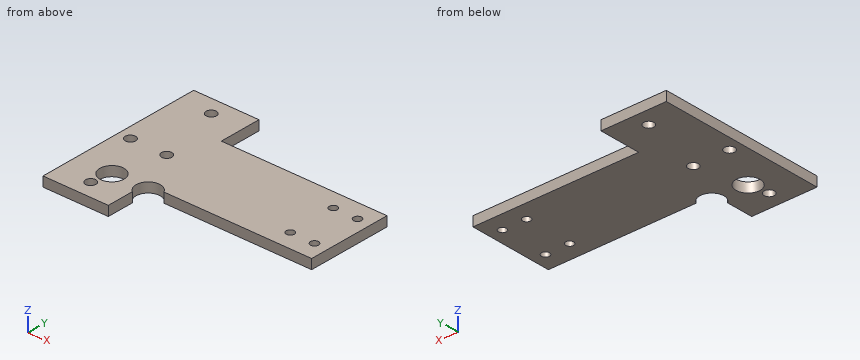
```python
from build123d import *

# Parameters (mm, degrees)
SKETCH_1_W          = 100
SKETCH_1_H          = 35
EXTRUDE_1_DEPTH     = 4
SKETCH_2_R          = 1.65
CUT_EXTRUDE_1_DEPTH = 107.023582282
SKETCH_4_R          = 2.15
CUT_EXTRUDE_3_DEPTH = 107.023582282
SKETCH_8_W          = 27
SKETCH_8_H          = 70
SKETCH_8_R          = 2.15
EXTRUDE_2_DEPTH     = 4
SKETCH_9_R          = 5
CUT_EXTRUDE_6_DEPTH = 4
SKETCH_10_R         = 1.65
CUT_EXTRUDE_7_DEPTH = 10
SKETCH_11_W         = 4.5
SKETCH_11_H         = 35
CUT_EXTRUDE_8_DEPTH = 10


with BuildPart() as part:
    # 草图1 → 凸台-拉伸1 (new body)
    with BuildSketch(Plane.XY):
        with Locations((50, -17.5)):
            Rectangle(SKETCH_1_W, SKETCH_1_H)
    extrude(amount=EXTRUDE_1_DEPTH)

    # 草图2 → 切除-拉伸1 (cut, through all)
    with BuildSketch(Plane.XY.offset(4)):
        with Locations((80, -7.5)):
            Circle(SKETCH_2_R)
        with Locations(Location((80, -27.5, 0), (0, 0, 180))):
            Circle(SKETCH_2_R)
    extrude(amount=-CUT_EXTRUDE_1_DEPTH, mode=Mode.SUBTRACT)

    # 草图4 → 切除-拉伸3 (cut, through all)
    with BuildSketch(Plane.XY.offset(4)):
        with Locations((5, -17.5)):
            Circle(SKETCH_4_R)
        with Locations((20, -17.5)):
            Circle(SKETCH_4_R)
    extrude(amount=-CUT_EXTRUDE_3_DEPTH, mode=Mode.SUBTRACT)

    # 草图8 → 凸台-拉伸2 (add)
    with BuildSketch(Plane.XY.offset(4)):
        with Locations((13.5, -17.5)):
            Rectangle(SKETCH_8_W, SKETCH_8_H)
        with Locations((13.5, 10.5)):
            Circle(SKETCH_8_R, mode=Mode.SUBTRACT)
        with Locations(Location((13.5, -45.5, 0), (0, 0, 180))):
            Circle(SKETCH_8_R, mode=Mode.SUBTRACT)
        with Locations((5, -17.5)):
            Circle(SKETCH_8_R, mode=Mode.SUBTRACT)
        with Locations((20, -17.5)):
            Circle(SKETCH_8_R, mode=Mode.SUBTRACT)
    extrude(amount=-EXTRUDE_2_DEPTH)

    # 草图9 → 切除-拉伸6 (cut)
    with BuildSketch(Plane.XY.offset(4)):
        with Locations((30, -37.34)):
            Circle(SKETCH_9_R)
        with Locations((15, -37.34)):
            Circle(SKETCH_9_R)
    extrude(amount=-CUT_EXTRUDE_6_DEPTH, mode=Mode.SUBTRACT)

    # 草图10 → 切除-拉伸7 (cut)
    with BuildSketch(Plane.XY.offset(4)):
        with Locations((90, -7.5)):
            Circle(SKETCH_10_R)
        with Locations((90, -27.5)):
            Circle(SKETCH_10_R)
    extrude(amount=-CUT_EXTRUDE_7_DEPTH, mode=Mode.SUBTRACT)

    # 草图11 → 切除-拉伸8 (cut)
    with BuildSketch(Plane.XY.offset(4)):
        with Locations((97.75, -17.5)):
            Rectangle(SKETCH_11_W, SKETCH_11_H)
    extrude(amount=-CUT_EXTRUDE_8_DEPTH, mode=Mode.SUBTRACT)


solid = part.part
```
Can you work these out from the model? Positions are in its coordinate system, mm. Round coordinates to 2 decimals unless told otherwise and drop trailing zeros. Loops run counter-clockwise (first coordinate to the right, second up) from the corner with the lowest first, then second, coordinate; pieces in that order, holes last. Notation, with made-up numbers: M -28.5,42 L 25.5,42 A31 ccw 25.5,70 Z; hole C 42,7 d4. An arc over 180 degrees is marked long. Answer as a JSON object with one key per item and string values. Group by question number.
Q1. Imagine slicing it at A-A, the plane x = 5. Please give me the cut outline in (y, z).
Q2. Imagine slicing it at D-D, the plane y = -45.5. Please give me the cut outline in (x, z).
Q3. Please list where these lines run through material, in increasing order: L1, parallel to Y at x = 80, z = 0.6; L2, parallel to X at y = -45.5, z = 0.85; L3, parallel to Y at x = 5, z = 1.95.
Q4. Will these pins go through, and if not, where does the flat tip stop? pin 1 (1.2 mm diameter, centred on x = 54, z = 1, fed in from -Y); pin 2 (3.5 mm diameter, centred on x = 13.5, y = 10.5, fed in from -Z); pin 3 (2 mm diameter, centred on y = 6.5, z = 2, fed in from +X); pin 4 (2 mm diameter, centred on x = 55, z = 1.5, fed in from +Y).
Q5. Imagine slicing it at B-B, the plane y = -18.5. Please give me the cut outline in (x, z).
Q6. Imagine slicing it at C-C, the plane z = 0.75. Count the separate pieces of the cut face and the enclosed holes in it, then the cut area to 3 significant figures.
Findings:
{
 "1": {"outline": "M -52.5,0 L -19.65,0 L -19.65,4 L -52.5,4 Z; M -15.35,0 L 17.5,0 L 17.5,4 L -15.35,4 Z"},
 "2": {"outline": "M 0,0 L 11.35,0 L 11.35,4 L 0,4 Z; M 15.65,0 L 27,0 L 27,4 L 15.65,4 Z"},
 "3": {"L1": "y = -35 to -29.15, -25.85 to -9.15, -5.85 to 0", "L2": "x = 0 to 11.35, 15.65 to 27", "L3": "y = -52.5 to -19.65, -15.35 to 17.5"},
 "4": {"pin 1": "stops at y = -35", "pin 2": "passes through", "pin 3": "stops at x = 27", "pin 4": "stops at y = 0"},
 "5": {"outline": "M 0,0 L 3.1,0 L 3.1,4 L 0,4 Z; M 6.9,0 L 18.1,0 L 18.1,4 L 6.9,4 Z; M 21.9,0 L 95.5,0 L 95.5,4 L 21.9,4 Z"},
 "6": {"separate pieces": "1", "enclosed holes": "9", "area": "4,090 mm2"}
}
